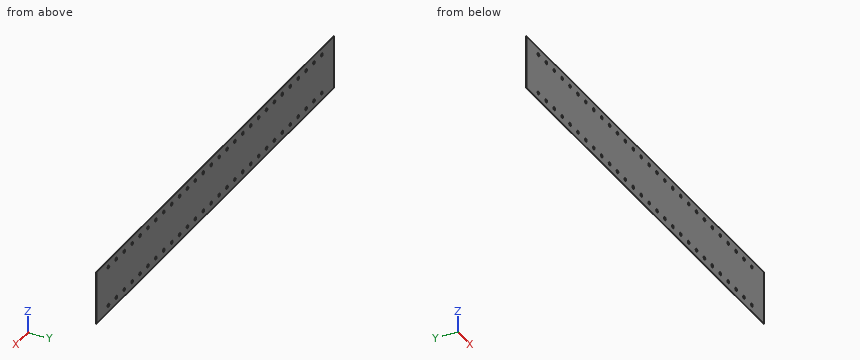
Autodesk Inventor part; units mm, degrees
ref_plane "YZ Plane" through (0, 0, 0) normal (1, 0, 0) x (0, 1, 0)
ref_plane "XZ Plane" through (0, 0, 0) normal (0, 1, 0) x (-1, 0, 0)
ref_plane "XY Plane" through (0, 0, 0) normal (0, 0, 1) x (1, 0, 0)
sketch "Skin Scheme" plane through (0, 0, 0) normal (0, 1, 0) x (-1, 0, 0)
  line L0 (756.5, -84.5) -> (-756.5, -84.5)
  line L1 (-756.5, -84.5) -> (-756.5, 84.5)
  line L2 (-756.5, 84.5) -> (756.5, 84.5)
  line L3 (756.5, 84.5) -> (756.5, -84.5)
  circle A0 centre (634.5, -62.5) radius 5
  circle A1 centre (587.5, -62.5) radius 5
  circle A2 centre (540.5, -62.5) radius 5
  circle A3 centre (493.5, -62.5) radius 5
  circle A4 centre (446.5, -62.5) radius 5
  circle A5 centre (399.5, -62.5) radius 5
  circle A6 centre (352.5, -62.5) radius 5
  circle A7 centre (305.5, -62.5) radius 5
  circle A8 centre (258.5, -62.5) radius 5
  circle A9 centre (211.5, -62.5) radius 5
  circle A10 centre (164.5, -62.5) radius 5
  circle A11 centre (117.5, -62.5) radius 5
  circle A12 centre (70.5, -62.5) radius 5
  circle A13 centre (23.5, -62.5) radius 5
  circle A14 centre (-23.5, -62.5) radius 5
  circle A15 centre (-70.5, -62.5) radius 5
  circle A16 centre (-117.5, -62.5) radius 5
  circle A17 centre (-164.5, -62.5) radius 5
  circle A18 centre (634.5, 62.5) radius 5
  circle A19 centre (587.5, 62.5) radius 5
  circle A20 centre (540.5, 62.5) radius 5
  circle A21 centre (493.5, 62.5) radius 5
  circle A22 centre (446.5, 62.5) radius 5
  circle A23 centre (399.5, 62.5) radius 5
  circle A24 centre (352.5, 62.5) radius 5
  circle A25 centre (305.5, 62.5) radius 5
  circle A26 centre (258.5, 62.5) radius 5
  circle A27 centre (211.5, 62.5) radius 5
  circle A28 centre (164.5, 62.5) radius 5
  circle A29 centre (117.5, 62.5) radius 5
  circle A30 centre (70.5, 62.5) radius 5
  circle A31 centre (23.5, 62.5) radius 5
  circle A32 centre (-23.5, 62.5) radius 5
  circle A33 centre (-70.5, 62.5) radius 5
  circle A34 centre (-117.5, 62.5) radius 5
  circle A35 centre (-164.5, 62.5) radius 5
  circle A36 centre (-211.5, -62.5) radius 5
  circle A37 centre (-211.5, 62.5) radius 5
  circle A38 centre (-258.5, -62.5) radius 5
  circle A39 centre (-258.5, 62.5) radius 5
  circle A40 centre (-305.5, -62.5) radius 5
  circle A41 centre (-305.5, 62.5) radius 5
  circle A42 centre (-352.5, -62.5) radius 5
  circle A43 centre (-352.5, 62.5) radius 5
  circle A44 centre (-399.5, -62.5) radius 5
  circle A45 centre (-399.5, 62.5) radius 5
  circle A46 centre (-446.5, -62.5) radius 5
  circle A47 centre (-446.5, 62.5) radius 5
  circle A48 centre (-493.5, -62.5) radius 5
  circle A49 centre (-493.5, 62.5) radius 5
  circle A50 centre (-540.5, -62.5) radius 5
  circle A51 centre (-540.5, 62.5) radius 5
  circle A52 centre (-587.5, -62.5) radius 5
  circle A53 centre (-587.5, 62.5) radius 5
  circle A54 centre (-634.5, -62.5) radius 5
  circle A55 centre (-634.5, 62.5) radius 5
  point P0 (0, 0)
  dimension "d0" = 1513
  dimension "d1" = 756.5
  dimension "d2" = 169
  dimension "d3" = 84.5
  dimension "d4" = 10
  dimension "d5" = 122
  dimension "d6" = 22
  dimension "d9" = 47
  dimension "d12" = 125
extrude "Skin Body" add sketch "Skin Scheme" along normal blind 1
sketch "End Cut Outline" plane through (0, 1, 0) normal (0, 1, 0) x (1, 0, 0)
  line L0 (-706.5, 94.5) -> (-766.5, 94.5)
  line L1 (-766.5, 94.5) -> (-766.5, -94.5)
  line L2 (-766.5, -94.5) -> (-706.5, -94.5)
  line L3 (-706.5, -94.5) -> (-706.5, 94.5)
  line L4 (756.5, 84.5) -> (-756.5, 84.5)
  line L5 (-756.5, -84.5) -> (756.5, -84.5)
  line L6 (-756.5, 84.5) -> (-756.5, -84.5)
  point P0 (0, 0)
  dimension "d19" = 10
  dimension "d20" = 10
  dimension "d21" = 10
  dimension "d22" = 50
extrude "End Cut" cut sketch "End Cut Outline" along normal through all both and the other way through all
mirror "End Cut Mirror" about plane through (0, 0, 0) normal (1, 0, 0) of "End Cut"
properties part number "Skin NPS 14 Internal" material "Rubber, Silicone"
Part model, mm, in its own coordinate system. Coordinates: 2 decimals unless noted, no trailing zeros.
(1) Pin check, flat tips, straight feed: pin 1 Ø8 at (x, z) = (-493.5, 62.5) entering from +Y; pin 2 Ø6 at (x, z) = (78.5, -12.5) entering from -Y. Stop position of each tip, or through.
Check sheet entries:
pin 1: passes through
pin 2: stops at y = 0
(2) Slice it at A-A, the plane y = 0.4. State how many separate pieces and enclosed holes the cut face has, and give its area (3 significant figures).
Check sheet entries:
separate pieces: 1
enclosed holes: 56
area: 234,000 mm2
(3) Probe L1, parallel to Z at x = -258.5, y = 0.75; L2, parallel to Z at x = -584, y = 0.3. List the from-to ranges inside material, lowest first.
Check sheet entries:
L1: z = -84.5 to -67.5, -57.5 to 57.5, 67.5 to 84.5
L2: z = -84.5 to -66.07, -58.93 to 58.93, 66.07 to 84.5
